```python
from build123d import *

# Parameters (mm, degrees)
F1_DEPTH = 203.2
F4_DEPTH = 102.6000000987
F5_T     = -3.175


with BuildPart() as f1:
    # F0 (on Top) → F1 (new body)
    with BuildSketch(Plane.XY):
        with BuildLine():
            ThreePointArc((-43.4231416653, -33.1147542783), (-25.3999999994, -25.3999999994), (-8.4143115766, -15.610339234))
            ThreePointArc((-8.4143115766, -15.610339234), (-2.2375332054, -8.8668389281), (0, 0))
            Line((0, 0), (-101.5999999975, 0))
            Line((-101.5999999975, 0), (-101.5999999975, -50.7999999987))
            ThreePointArc((-101.5999999975, -50.7999999987), (-72.2898591354, -42.6867133396), (-43.4231416653, -33.1147542783))
        make_face()
        with BuildLine():
            Line((-101.5999999975, 0), (0, 0))
            ThreePointArc((0, 0), (-2.2375332054, 8.8668389281), (-8.4143115766, 15.610339234))
            ThreePointArc((-8.4143115766, 15.610339234), (-25.3999999994, 25.3999999994), (-43.4231416653, 33.1147542783))
            ThreePointArc((-43.4231416654, 33.1147542783), (-72.2898591354, 42.6867133396), (-101.5999999975, 50.7999999987))
            Line((-101.5999999975, 50.7999999987), (-101.5999999975, 0))
        make_face()
    extrude(amount=F1_DEPTH)

    # F3 (on offset) → F4 (cut, up to face)
    with BuildSketch(Plane.XZ.offset(50.8)):
        with BuildLine():
            Line((0, 203.2), (-101.5999999975, 203.2))
            Line((-101.5999999975, 203.2), (-101.5999999975, 101.6))
            ThreePointArc((-101.5999999975, 101.6), (-79.0155935729, 89.5289612451), (-57.15, 76.2))
            ThreePointArc((-57.15, 76.2), (-40.6457692508, 64.2865384365), (-25.4, 50.8))
            ThreePointArc((-25.4, 50.8), (-14.8980769231, 38.8326923077), (-6.35, 25.4))
            ThreePointArc((-6.35, 25.4), (-1.6115585547, 13.0908603613), (0, 0))
            Line((0, 0), (0, 203.2))
        make_face()
    extrude(amount=-F4_DEPTH, mode=Mode.SUBTRACT)

    # F5
    f5_openings = [f1.faces().sort_by_distance(p)[0] for p in [
        (-60.726739, 0, 0),
    ]]
    offset(amount=F5_T, openings=f5_openings)


solid = f1.part
```
The listing builds one solid part. Answer for the finished solid, in the listing's coordinates (mm). A direction names the side the tool comes from. Give positions to 0.01 mm unless a question says otherwise; leave off trailing zeros. Order: outer loops, then holes, each group sorted by start corner. A loop starts at its lowest first (then second) coordinate and runs counter-clockwise, first axis right, second up.
1) For faces 1 (the face through (-3.236, 10.51, 11.108)), 2 (the face through (-78.64, -0.65, 85.65)), determine the directions among +Z, -Z, +X, -X, +Y, -Y from which every point of the face is accessible in a straight line to the end or side of a thin tool.
Reported:
face 1: +Z, -Z, +X, +Y
face 2: -Z
2) Given P1, Ø12, axis at x = -78, z = 77, coming from the +Y side; P2, Ø5, axis at y = -25.5, z = 44.5, coming from the +X side; P3, Ø3, axis at x = -79, y = -21.5, coming from the +Z side, each flat-ended and moving along its own axis, determine where each tip first touches the part or whether it passes through.
Reported:
P1: stops at y = 46.12
P2: stops at x = -20.78
P3: stops at z = 90.37
3) Find section B-B on x = -48.5. Write down the section's boundary in (y, z), then the cut area to 3 significant figures.
Reported:
outline: (-34.92, 0) - (-31.55, 0) - (-31.55, 66.33) - (31.55, 66.33) - (31.55, 0) - (34.92, 0) - (34.92, 70.27) - (-34.92, 70.27) - close
area: 721 mm2
4) Consider line 1 along X through (y, z) = (20, 70.5) (3 decimals); line 2 along X through (y, z) = (8, 77.5) (1 decimal); line 3 along Y through (x, z) = (-69.5, 60). Determine where each line is inside the solid, lowest interval first.
Reported:
line 1: x = -101.6 to -98.425, -54.335 to -48.823
line 2: x = -101.6 to -98.4, -65.1 to -59.2
line 3: y = -41.83 to -38.51, 38.51 to 41.83
5) Find section C-C on y = -43.5. Write down the section's boundary in (x, z) (3 decimals).
Reported:
outline: (-101.6, 0) - (-98.425, 0) - (-98.425, 96.436) arc R449.447 cw to (-86.421, 90.046) - (-86.421, 0) - (-74.988, 0) - (-74.988, 87.2) arc R452.622 ccw to (-101.6, 101.6) - close
6) Find section D-D on z = 11. Write down the section's boundary in (x, y) (3 decimals), then the cut area to 3 significant figures.
Reported:
outline: (-101.6, -50.8) arc R606.665 ccw to (-43.423, -33.115) arc R165.682 ccw to (-8.414, -15.61) arc R18.687 ccw to (-1.133, -6.407) - (-1.133, 6.407) arc R18.687 ccw to (-8.414, 15.61) arc R165.682 ccw to (-43.423, 33.115) arc R606.665 ccw to (-101.6, 50.8) - close; hole (-98.425, -46.719) arc R603.49 ccw to (-44.498, -30.127) arc R162.507 ccw to (-10.16, -12.958) arc R15.512 ccw to (-4.38, -5.995) - (-4.38, 5.995) arc R15.512 ccw to (-10.16, 12.958) arc R162.507 ccw to (-44.498, 30.127) arc R603.49 ccw to (-98.425, 46.719) - close
area: 1,040 mm2
7) Determine the mould class of faces 3 (the face through (-72.7, -42.81, 38.8)), 4 (the face through (-98.425, 1, 48)), 5 (the face through (-79.33, -0.71, 89.71)) for opening direction Y: pulls with the +Y half, pulls with the -Y half, needs draft (parallel to the pull), parting line crosses it, or undercut.
Reported:
face 3: pulls with the -Y half
face 4: undercut
face 5: needs draft
8) Find section A-A on z = 43.5. Write down the section's boundary in (x, y) (3 decimals).
Reported:
outline: (-101.6, -50.8) arc R606.665 ccw to (-43.423, -33.115) arc R165.682 ccw to (-18.613, -21.807) - (-18.613, 21.807) arc R165.682 ccw to (-43.423, 33.115) arc R606.665 ccw to (-101.6, 50.8) - close; hole (-98.425, -46.719) arc R603.49 ccw to (-44.498, -30.127) arc R162.507 ccw to (-22.815, -20.488) - (-22.815, 20.488) arc R162.507 ccw to (-44.498, 30.127) arc R603.49 ccw to (-98.425, 46.719) - close
